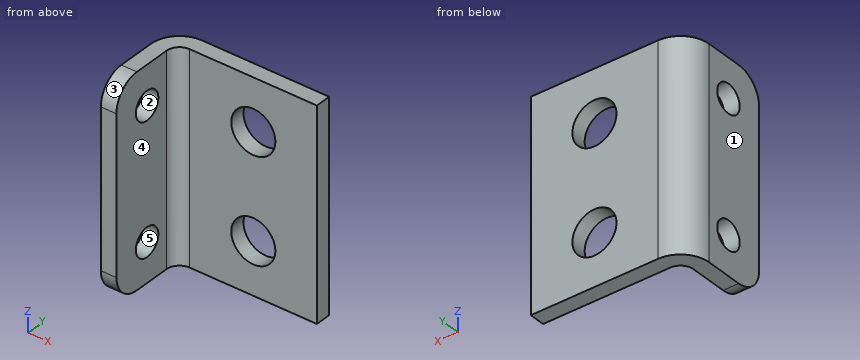
from build123d import *

# Parameters (mm, degrees)
F1_DEPTH = 40
F2_R     = 2.75
F4_DEPTH = 30.001
F3_R     = 4.25
F5_DEPTH = 3.001
F6_R     = 5


with BuildPart() as f1:
    # F0 (on Top) → F1 (new body)
    with BuildSketch(Plane.XY):
        with BuildLine():
            Line((0, 12.25), (0, 0))
            Line((0, 0), (3, 0))
            Line((3, 0), (3, 12.25))
            ThreePointArc((3, 12.25), (3.732233, 14.017767), (5.5, 14.75))
            Line((5.5, 14.75), (30, 14.75))
            Line((30, 14.75), (30, 17.75))
            Line((30, 17.75), (5.5, 17.75))
            ThreePointArc((5.5, 17.75), (1.610913, 16.139087), (0, 12.25))
        make_face()
    extrude(amount=F1_DEPTH)

    # F2 (on face) → F4 (cut, through all)
    with BuildSketch(Plane(origin=(0, 0, 0), x_dir=(0, -1, 0), z_dir=(-1, 0, 0))):
        with Locations((-7.5, 32.499999)):
            Circle(F2_R)
        with Locations((-7.5, 7.499999)):
            Circle(F2_R)
    extrude(amount=-F4_DEPTH, mode=Mode.SUBTRACT)

    # F3 (on face) → F5 (cut, through all)
    with BuildSketch(Plane.XZ.offset(-14.75)):
        with Locations((17.75, 10)):
            Circle(F3_R)
        with Locations((17.75, 30)):
            Circle(F3_R)
    extrude(amount=-F5_DEPTH, mode=Mode.SUBTRACT)

    # F6
    f6_edges = [f1.edges().sort_by_distance(p)[0] for p in [
        (1.5, 0, 40),
        (1.5, 0, 0),
    ]]
    fillet(f6_edges, radius=F6_R)


solid = f1.part
Read the model definition and answer for the solid it produces. Units are mm, in the model's axes. Face numbers are marked on the shaded views. A direction names the side the tool comes from. Coordinates: 2 decimals unless noted, no trailing zeros. Order: outer loops, then holes, each group sorted by start corner. A loop starts at its lowest first (then second) coordinate and runs counter-clockwise, first axis right, second up. Notation, with made-up numbers: M 21,43.25 L 44,43.25 A34 ccw 44,80.25 Z; hole C 15.25,54.25 d2. An arc over 180 degrees is marked long. Put each result on its own line as item: value. Start each with the question number.
Item 1: The mould has two halves that part along Z. Classify the marked faces 1, 2 and 3: +Z half, -Z half, draft (parallel to the pull), parting line (faces both ways), or undercut.
Item 2: Section A-A, the plane x = 17.75 is taken. Determine the outline of the cut face in (y, z).
Item 3: Section D-D, the plane z = 25 is taken. Determine the outline of the cut face in (x, y), plus the area to 3 significant figures.
Item 4: Section C-C, the plane y = 9 is taken. Determine the outline of the cut face in (x, z), plus the area to 3 significant figures.
Item 5: For the marked faces 4 and 5, determine the directions among +Z, -Z, +X, -X, +Y, -Y from which every point of the face is accessible in a straight line to the end or side of a thin tool.
Item 6: Given pin 1 Ø7 at (x, z) = (17.75, 10) entering from -Y; pin 2 Ø5 at (x, z) = (15, 9) entering from -Y; pin 3 Ø10 at (y, z) = (3, 16.5) entering from +X, each flat-ended and moving along its own axis, determine where each tip first touches the part or whether it passes through.
Item 7: Consider probe 1 along Z at (x, y) = (17.75, 16.4); probe 2 along Z at (x, y) = (2.3, 7.5); probe 3 along Y at (x, z) = (10.25, 18). Determine where each line is inside the solid, lowest interval first. Write a range as [from, to].
Item 8: Section B-B, the plane z = 32.5 is taken. Determine the outline of the cut face in (x, y), plus the area to 3 significant figures.
Computed:
1. face 1: draft
1. face 2: undercut
1. face 3: +Z half
2. outline: M 14.75,0 L 17.75,0 L 17.75,5.75 L 14.75,5.75 Z; M 14.75,14.25 L 17.75,14.25 L 17.75,25.75 L 14.75,25.75 Z; M 14.75,34.25 L 17.75,34.25 L 17.75,40 L 14.75,40 Z
3. outline: M 0,0 L 3,0 L 3,12.25 A2.5 cw 5.5,14.75 L 30,14.75 L 30,17.75 L 5.5,17.75 A5.5 ccw 0,12.25 Z
3. area: 129 mm2
4. outline: M 0,0 L 3,0 L 3,5.2 L 0,5.2 Z; M 0,9.8 L 3,9.8 L 3,30.2 L 0,30.2 Z; M 0,34.8 L 3,34.8 L 3,40 L 0,40 Z
4. area: 92.3 mm2
5. face 4: +Z, -Z, +X, -Y
5. face 5: +X, -X
6. pin 1: passes through
6. pin 2: stops at y = 14.75
6. pin 3: stops at x = 3
7. probe 1: z = [0, 5.75], [14.25, 25.75], [34.25, 40]
7. probe 2: z = [0, 4.75], [10.25, 29.75], [35.25, 40]
7. probe 3: y = [14.75, 17.75]
8. outline: M 0,0 L 3,0 L 3,4.75 L 0,4.75 Z; M 0,10.25 L 3,10.25 L 3,12.25 A2.5 cw 5.5,14.75 L 14.31,14.75 L 14.31,17.75 L 5.5,17.75 A5.5 ccw 0,12.25 Z; M 21.19,14.75 L 30,14.75 L 30,17.75 L 21.19,17.75 Z
8. area: 92.0 mm2
